Check sheet for the drawn part. Datum: minimum x, y, z corner. Units: mm. Coordinates: 2 decimals unless noted, no trailing zeros. Order: outer loops, then holes, each group sorted by start corner. A loop starts at its lowest first (then second) coordinate and runs counter-clockwise, first axis right, second up.
1. Gauge pin test, flat end, axial feed: pin 1 Ø5 at (y, z) = (78, 5) entering from -X. Record the tip position at first contact, or that the pin passes through.
2. Thickness scan on line 1 (X direction, y = 137.5, z = 9.75); line 2 (Y direction, x = 184, z = 5). Record the ranges inside material, lowest first.
3. Cross-section at B-B (z = 6.25). Enter the section's corners in (x, y), then the cut area to 3 significant figures.
4. Cross-section at A-A (y = 121). Enter the section's corners in (x, z).
5. Cross-section at C-C (x = 182). Enter the section's corners in (y, z).
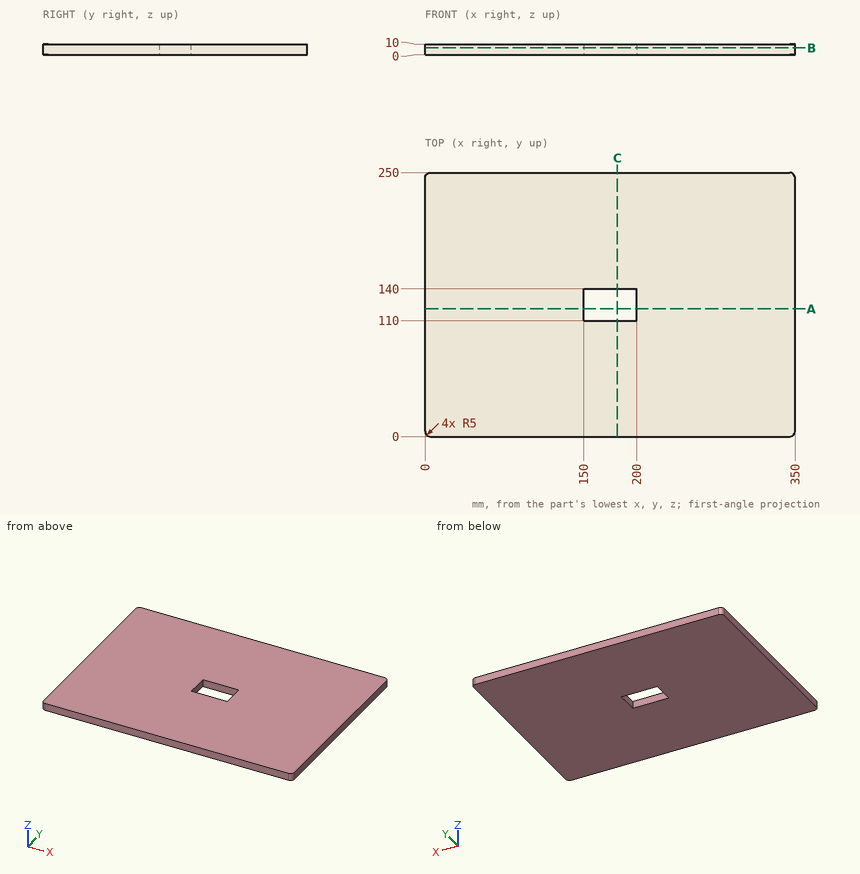
Data:
1. pin 1: stops at x = 0
2. line 1: x = 0 to 150, 200 to 350
2. line 2: y = 0 to 110, 140 to 250
3. outline: (0, 5) arc R5 ccw to (5, 0) - (345, 0) arc R5 ccw to (350, 5) - (350, 245) arc R5 ccw to (345, 250) - (5, 250) arc R5 ccw to (0, 245) - close; hole (150, 110) - (200, 110) - (200, 140) - (150, 140) - close
3. area: 86,000 mm2
4. outline: (0, 0) - (150, 0) - (150, 10) - (0, 10) - close; (200, 0) - (350, 0) - (350, 10) - (200, 10) - close
5. outline: (0, 0) - (110, 0) - (110, 10) - (0, 10) - close; (140, 0) - (250, 0) - (250, 10) - (140, 10) - close
